Verification items for this drawing (mm, ordinates from the low corner). A direction names the side the tool comes from. Round coordinates to 2 decimals unless told otherwise and drop trailing zeros. Write each loop counter-clockwise with the first axis right and the second up, starting at its lowest first coordinate (ties: lowest second). Pieces come first, ordered by that corner, then holes. Notation, with made-up numbers: M 88,-27 L 111,-27 A25 cw 111,4 Z; hole C -31.75,30.25 d3. An arc over 180 degrees is marked long. Write each question's results on one line, items separated by ' | '.
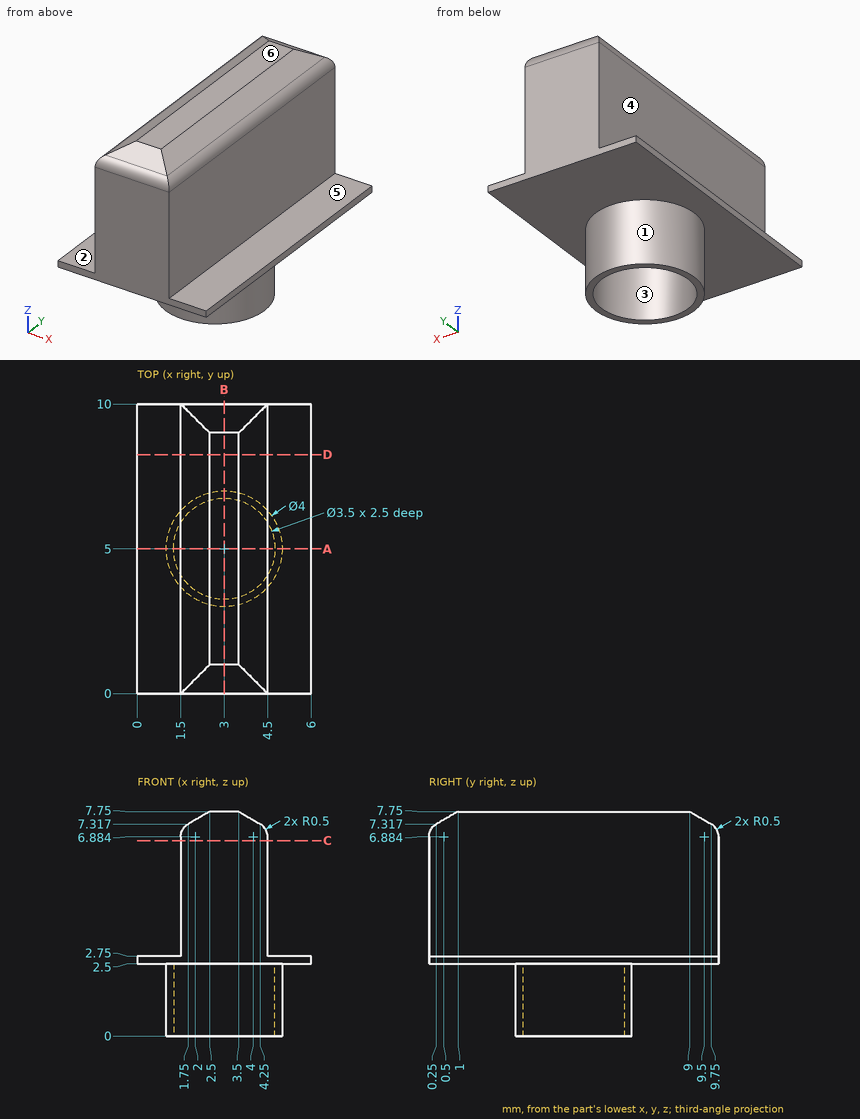
1) Depth check by flat-ended pin: P1, Ø3, axis at y = 4, z = 5.5, coming from the -X side; P2, Ø1.2, axis at x = 0.5, y = 7.5, coming from the +Z side; P3, Ø1.5, axis at y = 7, z = 1.5, coming from the -X side. Enter the tip coordinate at first touch or a pass-through.
Calculated:
P1: stops at x = 1.5 | P2: stops at z = 2.75 | P3: stops at x = 1.44
2) Sectioned sample at C-C, the plane z = 6.75. Record the cut outline in (x, y), and give its area (3 significant figures).
Calculated:
outline: M 1.5,0 L 4.5,0 L 4.5,10 L 1.5,10 Z | area: 30.0 mm²
3) Draft check along Y on the marked faces 1, 2 and 3. Enter one of: pulls with the +Y half, pulls with the -Y half, needs draft (parallel to the pull), parting line crosses it, or undercut.
Calculated:
face 1: parting line crosses it | face 2: needs draft | face 3: undercut
4) Sectioned sample at D-D, the plane y = 8.25. Record the cut outline in (x, z), and give its area (3 significant figures).
Calculated:
outline: M 0,2.5 L 6,2.5 L 6,2.75 L 4.5,2.75 L 4.5,6.88 A0.5 ccw 4.25,7.32 L 3.5,7.75 L 2.5,7.75 L 1.75,7.32 A0.5 ccw 1.5,6.88 L 1.5,2.75 L 0,2.75 Z | area: 15.9 mm²
5) Sectioned sample at A-A, the plane y = 5. Record the cut outline in (x, z).
Calculated:
outline: M 0,2.5 L 1,2.5 L 1,0 L 1.25,0 L 1.25,2.5 L 4.75,2.5 L 4.75,0 L 5,0 L 5,2.5 L 6,2.5 L 6,2.75 L 4.5,2.75 L 4.5,6.88 A0.5 ccw 4.25,7.32 L 3.5,7.75 L 2.5,7.75 L 1.75,7.32 A0.5 ccw 1.5,6.88 L 1.5,2.75 L 0,2.75 Z
6) Access from +Z, -Z, +X, -X, +Y, -Y to the whole of each face (thin tool, end or side, straight path). Record for the marked faces 4, 5 and 6.
Calculated:
face 4: +Z, -X, +Y, -Y | face 5: +Z, +X, +Y, -Y | face 6: +Z, +X, -X, +Y, -Y
7) Material ranges on line 1 (Y direction, x = 3, z = 1.1); line 2 (Z direction, x = 1.15, y = 3); line 3 (X direction, y = 9.25, z = 4), recorded low to high. Write a range as [from, to].
Calculated:
line 1: y = [3, 3.25], [6.75, 7] | line 2: z = [2.5, 2.75] | line 3: x = [1.5, 4.5]
8) Sectioned sample at B-B, the plane x = 3. Record the cut outline in (y, z).
Calculated:
outline: M 0,2.5 L 3,2.5 L 3,0 L 3.25,0 L 3.25,2.5 L 6.75,2.5 L 6.75,0 L 7,0 L 7,2.5 L 10,2.5 L 10,6.88 A0.5 ccw 9.75,7.32 L 9,7.75 L 1,7.75 L 0.25,7.32 A0.5 ccw 0,6.88 Z
